from build123d import *

# Parameters (mm, degrees)
EXTRUDE_1_DEPTH     = 5
SKETCH_2_W          = 12.2
SKETCH_2_H          = 22.5
CUT_EXTRUDE_1_DEPTH = 108.819293264


with BuildPart() as part:
    # ｽｹｯﾁ1 → ﾎﾞｽ - 押し出し1 (new body)
    with BuildSketch(Plane.XY):
        with BuildLine():
            Line((35, 100), (-35, 100))
            Line((-35, 100), (-35, 19.364916731))
            ThreePointArc((-35, 19.364916731), (0, -40), (35, 19.364916731))
            Line((35, 19.364916731), (35, 100))
        make_face()
    extrude(amount=EXTRUDE_1_DEPTH)

    # ｽｹｯﾁ2 → ｶｯﾄ - 押し出し1 (cut, through all)
    with BuildSketch(Plane.XY.offset(5)):
        with Locations((-36, 72.689802684)):
            Rectangle(SKETCH_2_W, SKETCH_2_H)
    extrude(amount=-CUT_EXTRUDE_1_DEPTH, mode=Mode.SUBTRACT)


solid = part.part
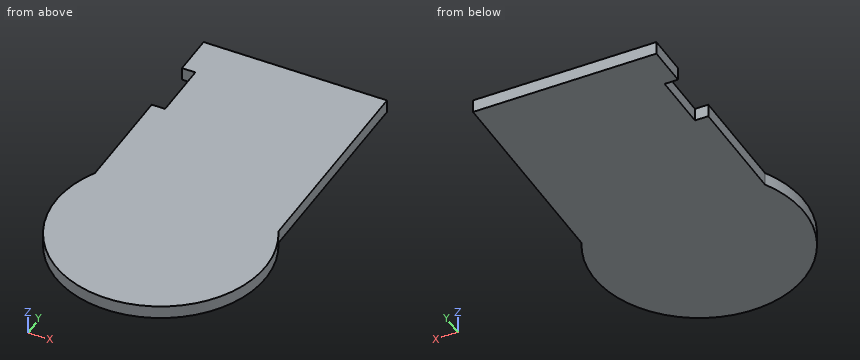
Verification items for the finished model (mm, model axes). Give positions to 0.01 mm unless a question says otherwise; leave off trailing zeros. Loops run counter-clockwise (first coordinate to the right, second up) from the corner with the lowest first, then second, coordinate; pieces in that order, holes last.
1. Cross-section at B-B on y = 38. Record the cut outline in (x, z).
Derived:
outline: (-35, 0) - (35, 0) - (35, 5) - (-35, 5) - close
2. Cross-section at C-C on x = -19.5. Record the cut outline in (y, z).
Derived:
outline: (-34.92, 0) - (100, 0) - (100, 5) - (-34.92, 5) - close
3. Material ranges on probe 1 along X at (y, z) = (1, 0.7); probe 2 along X at (y, z) = (54, 3.3); probe 3 along Y at (x, z) = (0, 3.2), recorded low to high.
Derived:
probe 1: x = -39.99 to 39.99
probe 2: x = -35 to 35
probe 3: y = -40 to 100
4. Go/stop test with flat-tipped pins: P1, Ø2, axis at y = 55, z = 4, coming from the +X side; P2, Ø2, axis at x = -17, z = 3, coming from the -Y side; P3, Ø8, axis at x = -26.5, y = -24.5, coming from the -Z side; P4, Ø3, axis at y = -16, z = 1, coming from the +X side. Record where each tip stops, or that it passes through.
Derived:
P1: stops at x = 35
P2: stops at y = -36.66
P3: stops at z = 0
P4: stops at x = 37.28
5. Cross-section at A-A on z = 3.4. Record the cut outline in (x, y), and give its area (3 significant figures).
Derived:
outline: (-35, 19.36) arc R40 ccw (long way) to (35, 19.36) - (35, 100) - (-35, 100) - (-35, 83.94) - (-29.9, 83.94) - (-29.9, 61.44) - (-35, 61.44) - close
area: 9,530 mm2
